Autodesk Inventor part; units mm, degrees
ref_plane "YZ Plane" through (0, 0, 0) normal (1, 0, 0) x (0, 1, 0)
ref_plane "XZ Plane" through (0, 0, 0) normal (0, 1, 0) x (-1, 0, 0)
ref_plane "XY Plane" through (0, 0, 0) normal (0, 0, 1) x (1, 0, 0)
sketch "Sketch1" plane through (0, 0, 0) normal (1, 0, 0) x (0, 1, 0)
  circle A0 centre (0, 0) radius 40
  dimension "d0" = 80
extrude "Extrusion1" add sketch "Sketch1" along normal blind 15
sketch "Sketch2" plane through (0, 0, 0) normal (-1, 0, 0) x (0, 0, 1)
  circle A0 centre (0, 0) radius 25
  circle A1 centre (0, 0) radius 40
  dimension "d3" = 50
extrude "Extrusion2" add sketch "Sketch2" along normal blind 25 contours A0
sketch "Sketch3" plane through (-25, 0, 0) normal (-1, 0, 0) x (0, 0, 1)
  circle A0 centre (0, 0) radius 20
  circle A1 centre (0, 0) radius 25
  dimension "d6" = 40
extrude "Extrusion3" add sketch "Sketch3" along normal blind 120 contours A0
sketch "Sketch4" plane through (-145, 0, 0) normal (-1, 0, 0) x (0, 0, 1)
  circle A0 centre (0, 0) radius 15
  circle A1 centre (0, 0) radius 20
  dimension "d9" = 30
extrude "Extrusion4" add sketch "Sketch4" along normal blind 15 contours A0
sketch "Sketch5" plane through (-160, 0, 0) normal (-1, 0, 0) x (0, 0, 1)
  line L0 (-10, 10) -> (10, 10)
  line L1 (10, 10) -> (10, -10)
  line L2 (10, -10) -> (-10, -10)
  line L3 (-10, -10) -> (-10, 10)
  point P0 (0, 0)
  dimension "d12" = 20
  dimension "d13" = 20
  dimension "d14" = 10
  dimension "d15" = 10
extrude "Extrusion5" add sketch "Sketch5" along normal blind 20
sketch "Sketch6" plane through (15, 0, 0) normal (1, 0, 0) x (0, 0, -1)
  line L0 (-15, 15) -> (15, 15)
  line L1 (15, 15) -> (15, -15)
  line L2 (15, -15) -> (-15, -15)
  line L3 (-15, -15) -> (-15, 15)
  point P0 (0, 0)
  point P1 (-15, 0)
  point P2 (0, 15)
  dimension "d18" = 30
  dimension "d19" = 30
  dimension "d20" = 15
  dimension "d21" = 15
extrude "Extrusion6" cut sketch "Sketch6" against normal blind 5
sketch "Sketch7" plane through (15, 0, 0) normal (1, 0, 0) x (0, 0, -1)
  circle A0 centre (0, 32) radius 4
  circle A1 centre (32, 0) radius 4
  circle A2 centre (-32, 0) radius 4
  circle A3 centre (0, -32) radius 4
  circle A4 centre (0, 0) radius 32 construction
  circle A5 centre (0, 0) radius 40
  dimension "d24" = 64
  dimension "d25" = 8
extrude "Extrusion7" cut sketch "Sketch7" against normal through all contours A0 | A1 | A2 | A3
properties part number "DRIVE SHAFT"
The model under review builds one solid part; all positions refer to its coordinate system, in mm. A direction names the side the tool comes from. Round coordinates to 2 decimals unless told otherwise and drop trailing zeros. Loops run counter-clockwise (first coordinate to the right, second up) from the corner with the lowest first, then second, coordinate; pieces in that order, holes last. Notation, with made-up numbers: (84, -26.75) -> (142, -26.75) arc R16 ccw to (142, -12.75) -> close; hole circle Ø6 at (-25.75, 69.5). An arc over 180 degrees is marked (long way). One line per question, with ' | ' between items. Start each with the question number.
Item 1: Draft analysis for pull direction Y (two halves, no side actions). For faces 4 (the face through (7.605, -28.034, 0.521)), 5 (the face through (15, 17, 1)), 6 (the face through (-152.395, -0.66, -14.985)), 7 (the face through (10, 0, 0)), state which applies: +Y half, -Y half, draft (parallel to the pull), parting line (faces both ways), or undercut.
Item 2: Wall thickness on line 1 along X through (y, z) = (-10.5, 35.5); line 2 along Z through (x, y) = (-158.5, 1); line 3 along X through (y, z) = (11.5, -21): over which ranges is each line inside the solid? List them lowest first. Write a range as [from, to].
Item 3: Add section C-C, the plane z = -32. Write out the cut boundary in (x, y).
Item 4: Add section A-A, the plane z = 0. Count the separate pieces of the cut face and the enclosed holes in it, then the cut area to 3 significant figures.
Item 5: Machinability: for faces 1 (the face through (-84.16, 19.524, -4.336)), 2 (the face through (-170, 0, 10)), 3 (the face through (13, 0, 15)), which of the approach directions +Z, -Z, +X, -X, +Y, -Y give a long, thin tool a straight path to every point of the face, cutting with its end or side? Answer none if there is none.
Item 6: For pin 1 (5.5 mm diameter, centred on x = 12.5, z = 5.5, fed in from -Y); pin 2 (10 mm diameter, centred on x = -117, y = 3.5, fed in from +Z); pin 3 (5 mm diameter, centred on y = 0, z = -32, fed in from -X); pin 4 (5 mm diameter, centred on x = -11, z = -16, fed in from -Y), all flat-tipped, find the tip position at first contact; note any pin that passes through.
Return value:
1) face 4: undercut | face 5: draft | face 6: parting line | face 7: undercut
2) line 1: x = [0, 15] | line 2: z = [-14.97, 14.97] | line 3: x = [-25, 15]
3) outline: (0, -24) -> (15, -24) -> (15, -4) -> (0, -4) -> close; (0, 4) -> (15, 4) -> (15, 24) -> (0, 24) -> close
4) separate pieces: 3 | enclosed holes: 0 | area: 7,710 mm2
5) face 1: -X | face 2: +Z, -X, +Y, -Y | face 3: +X
6) pin 1: stops at y = -39.91 | pin 2: stops at z = 20 | pin 3: passes through | pin 4: stops at y = -21.04
